Geometry check sheet. Reference: drawing and pictorial views, mm from the part's lowest x, y, z. Give positions to 0.01 mm unless a question says otherwise; leave off trailing zeros. Write each loop counter-clockwise with the first axis right and the second up, starting at its lowest first coordinate (ties: lowest second). Pieces come first, ordered by that corner, then holes.
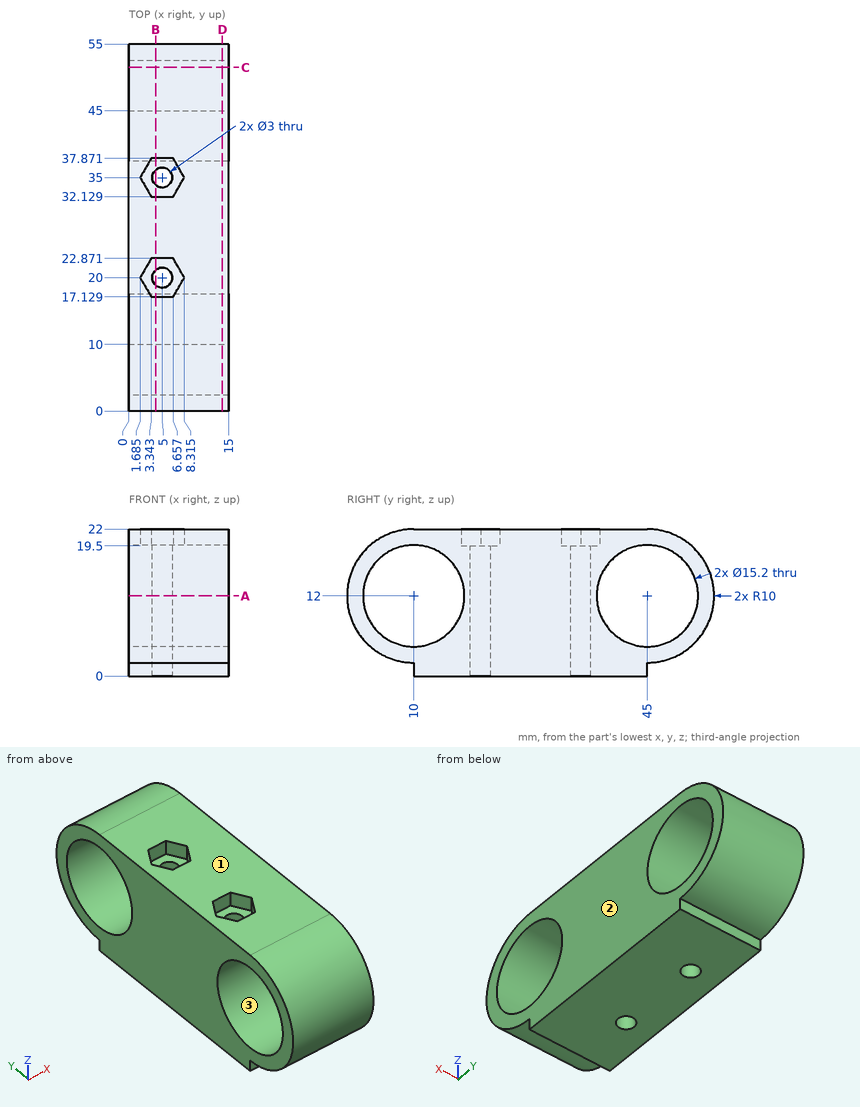
Item 1: Release check for a two-part mould opening along Z. For the marked faces 1, 2 and 3 record: released by +Z, released by -Z, zero draft, split by the parting line, or undercut.
Answer key:
face 1: released by +Z
face 2: zero draft
face 3: undercut
Item 2: Scan lines: line 1 along X through (y, z) = (35, 12.75); line 2 along Y through (x, z) = (1.5, 7.25) (1 decimal); line 3 along Y through (x, z) = (5, 15). Record each from-to range of solid material in increasing order.
Answer key:
line 1: x = 0 to 3.5, 6.5 to 15
line 2: y = 1.2 to 4.1, 15.9 to 39.1, 50.9 to 53.8
line 3: y = 0.46 to 3.02, 16.98 to 18.5, 21.5 to 33.5, 36.5 to 38.02, 51.98 to 54.54
Item 3: Sectioned sample at C-C on y = 51.5. Record the cut outline in (x, z).
Answer key:
outline: (0, 4.4) - (15, 4.4) - (15, 8.06) - (0, 8.06) - close; (0, 15.94) - (15, 15.94) - (15, 19.6) - (0, 19.6) - close
Item 4: Sectioned sample at D-D on x = 14. Record the cut outline in (y, z), then the cut area to 3 significant figures.
Answer key:
outline: (10, 0) - (45, 0) - (45, 2) arc R10 ccw to (45, 22) - (10, 22) arc R10 ccw to (10, 2) - close; hole circle Ø15.2 at (10, 12); hole circle Ø15.2 at (45, 12)
area: 721 mm2
Item 5: Depth check by flat-ended pin: pin 1 (8 mm diameter, centred on x = 2.5, z = 17.5, fed in from +Y); pin 2 (1.6 mm diameter, centred on x = 4, z = 1, fed in from -Y); pin 3 (1.6 mm diameter, centred on x = 5.5, z = 1, fed in from +Y). Enter the tip coordinate at first touch or a pass-through.
Answer key:
pin 1: stops at y = 54.89
pin 2: stops at y = 10
pin 3: stops at y = 45
Item 6: Sectioned sample at B-B on x = 4. Record the cut outline in (y, z).
Answer key:
outline: (10, 0) - (18.88, 0) - (18.88, 19.5) - (17.13, 19.5) - (17.13, 22) - (10, 22) arc R10 ccw to (10, 2) - close; (21.12, 0) - (33.88, 0) - (33.88, 19.5) - (32.13, 19.5) - (32.13, 22) - (22.87, 22) - (22.87, 19.5) - (21.12, 19.5) - close; (36.12, 0) - (45, 0) - (45, 2) arc R10 ccw to (45, 22) - (37.87, 22) - (37.87, 19.5) - (36.12, 19.5) - close; hole circle Ø15.2 at (10, 12); hole circle Ø15.2 at (45, 12)
Item 7: Sectioned sample at A-A on z = 12. Record the cut outline in (x, y).
Answer key:
outline: (0, 0) - (15, 0) - (15, 2.4) - (0, 2.4) - close; (0, 17.6) - (15, 17.6) - (15, 37.4) - (0, 37.4) - close; (0, 52.6) - (15, 52.6) - (15, 55) - (0, 55) - close; hole circle Ø3 at (5, 20); hole circle Ø3 at (5, 35)
